Design review of the part built by this model. Coordinates are the model's own, in mm. Face numbers are marked on the shaded views. A direction names the side the tool comes from. Give positions to 0.01 mm unless a question says otherwise; leave off trailing zeros. Order: outer loops, then holes, each group sorted by start corner. A loop starts at its lowest first (then second) coordinate and runs counter-clockwise, first axis right, second up. Notation, with made-up numbers: (50.5, 27) -> (89.5, 27) arc R26 ccw to (89.5, 49) -> close; hole circle Ø9 at (32.5, 26.5). An arc over 180 degrees is marked (long way). One line per item, written item: value. Start each with the question number.
1) Tool access review of the marked faces 1 and 2: name each direction out of +Z, -Z, +X, -X, +Y, -Y from which nothing blocks a thin tool from reaching the whole face with its end or side.
2) Consider section A-A (y = 1.5). State the section outline as (x, z) points.
3) Consider section B-B (y = 6.5). State the section outline as (x, z) points, plus the area to 3 significant figures.
4) For pin 1 (3 mm diameter, centred on y = 5, z = -10.5, fed in from -X); pin 2 (3 mm diameter, centred on y = 3, z = -8, fed in from -X), all flat-tipped, find the tip position at first contact; note any pin that passes through.
5) The part is to be moulded in two halves that separate along X. For the marked faces 3, 4, 5 and 6, say which applies: released by +X, released by -X, zero draft, split by the parting line, or undercut.
6) Wall thickness on line 1 along Y through (x, z) = (-53.5, -10.25); line 2 along Y through (x, z) = (-57.25, -22.5); line 3 along Z through (x, y) = (-52.75, 1.75): over which ranges is each line inside the solid? List them lowest first. Write a range as from..to.
from build123d import *

# Parameters (mm, degrees)
SZKIC1_R                    = 9
SZKIC1_R_2                  = 5.477333333
DODANIE_WYCI_GNI_CIE1_DEPTH = 8
SZKIC1_3_R                  = 11
SZKIC1_3_R_2                = 9
DODANIE_WYCI_GNI_CIE2_DEPTH = 7
SZKIC1_4_R                  = 11.95
SZKIC1_4_R_2                = 11
DODANIE_WYCI_GNI_CIE3_DEPTH = 3
DODANIE_WYCI_GNI_CIE4_START = -3
SZKIC1_5_R                  = 11.95
SZKIC1_5_R_2                = 1.65
SZKIC1_5_R_3                = 11
SZKIC1_5_R_4                = 9
SZKIC1_5_R_5                = 5.477333333
DODANIE_WYCI_GNI_CIE4_DEPTH = 3
SZKIC2_R                    = 8.25
WYTNIJ_WYCI_GNI_CIE1_DEPTH  = 5
SFAZOWANIE1_SIZE            = 1.2
DODANIE_WYCI_GNI_CIE5_START = 17
SZKIC3_R                    = 1.65
DODANIE_WYCI_GNI_CIE5_DEPTH = 17
ZAOKR_GLENIE1_R             = 10
ZAOKR_GLENIE2_R             = 4
SFAZOWANIE2_SIZE            = 2
WYTNIJ_WYCI_GNI_CIE3_DEPTH  = 81.474279011


# Some blends are built 0.0001 mm under size
with BuildPart() as part:
    # Szkic1 → Dodanie-wyciągnięcie1 (new body)
    with BuildSketch(Plane(origin=(0, 0, 0), x_dir=(1, 0, 0), z_dir=(0, 1, 0))):
        with Locations(Location((-48.017326928, 15.231452718, 0), (0, 0, 270))):
            Circle(SZKIC1_R)
        with Locations(Location((-48.017326928, 15.231452718, 0), (0, 0, 270))):
            Circle(SZKIC1_R_2, mode=Mode.SUBTRACT)
    extrude(amount=DODANIE_WYCI_GNI_CIE1_DEPTH)

    # Szkic1<3> → Dodanie-wyciągnięcie2 (add)
    with BuildSketch(Plane(origin=(0, 0, 0), x_dir=(1, 0, 0), z_dir=(0, 1, 0))):
        with Locations(Location((-48.017326928, 15.231452718, 0), (0, 0, 270))):
            Circle(SZKIC1_3_R)
        with Locations(Location((-48.017326928, 15.231452718, 0), (0, 0, 270))):
            Circle(SZKIC1_3_R_2, mode=Mode.SUBTRACT)
    extrude(amount=DODANIE_WYCI_GNI_CIE2_DEPTH)

    # Szkic1<4> → Dodanie-wyciągnięcie3 (add)
    with BuildSketch(Plane(origin=(0, 0, 0), x_dir=(1, 0, 0), z_dir=(0, 1, 0))):
        with Locations(Location((-48.017326928, 15.231452718, 0), (0, 0, 270))):
            Circle(SZKIC1_4_R)
        with Locations(Location((-48.017326928, 15.231452718, 0), (0, 0, 270))):
            Circle(SZKIC1_4_R_2, mode=Mode.SUBTRACT)
    extrude(amount=DODANIE_WYCI_GNI_CIE3_DEPTH)

    # Szkic1<5> → Dodanie-wyciągnięcie4 (add)
    # profile 1 of 4: a face of its own
    with BuildSketch(Plane(origin=(0, 0, 0), x_dir=(1, 0, 0), z_dir=(0, 1, 0)).offset(DODANIE_WYCI_GNI_CIE4_START)):
        with BuildLine():
            Line((-69.017326928, 26.22592553), (-69.017326928, 4.236979905))
            ThreePointArc((-69.017326928, 4.236979905), (-67.978820752, -1.151729035), (-65.012060165, -5.768547282))
            Line((-65.012060165, -5.768547282), (-50.017326928, -5.768547282))
            Line((-50.017326928, -5.768547282), (-30.833560744, -5.768547282))
            Line((-30.833560744, -5.768547282), (-26.817326928, -1.752313466))
            Line((-26.817326928, -1.752313466), (-26.817326928, 32.215218902))
            Line((-26.817326928, 32.215218902), (-30.833560744, 36.231452718))
            Line((-30.833560744, 36.231452718), (-50.017326928, 36.231452718))
            Line((-50.017326928, 36.231452718), (-65.012060165, 36.231452718))
            ThreePointArc((-65.012060165, 36.231452718), (-67.978820752, 31.61463447), (-69.017326928, 26.22592553))
        make_face()
        with Locations(Location((-48.017326928, 15.231452718, 0), (0, 0, 270))):
            Circle(SZKIC1_5_R, mode=Mode.SUBTRACT)
        with Locations(Location((-63.517326928, -0.268547282, 0), (0, 0, 270))):
            Circle(SZKIC1_5_R_2, mode=Mode.SUBTRACT)
        with Locations(Location((-32.517326928, -0.268547282, 0), (0, 0, 270))):
            Circle(SZKIC1_5_R_2, mode=Mode.SUBTRACT)
        with Locations(Location((-32.517326928, 30.731452718, 0), (0, 0, 270))):
            Circle(SZKIC1_5_R_2, mode=Mode.SUBTRACT)
        with Locations(Location((-63.517326928, 30.731452718, 0), (0, 0, 270))):
            Circle(SZKIC1_5_R_2, mode=Mode.SUBTRACT)
    # profile 2 of 4: a face of its own
    with BuildSketch(Plane(origin=(0, 0, 0), x_dir=(1, 0, 0), z_dir=(0, 1, 0)).offset(DODANIE_WYCI_GNI_CIE4_START)):
        with Locations(Location((-48.017326928, 15.231452718, 0), (0, 0, 270))):
            Circle(SZKIC1_5_R)
        with Locations(Location((-48.017326928, 15.231452718, 0), (0, 0, 270))):
            Circle(SZKIC1_5_R_3, mode=Mode.SUBTRACT)
    # profile 3 of 4: a face of its own
    with BuildSketch(Plane(origin=(0, 0, 0), x_dir=(1, 0, 0), z_dir=(0, 1, 0)).offset(DODANIE_WYCI_GNI_CIE4_START)):
        with Locations(Location((-48.017326928, 15.231452718, 0), (0, 0, 270))):
            Circle(SZKIC1_5_R_3)
        with Locations(Location((-48.017326928, 15.231452718, 0), (0, 0, 270))):
            Circle(SZKIC1_5_R_4, mode=Mode.SUBTRACT)
    # profile 4 of 4: a face of its own
    with BuildSketch(Plane(origin=(0, 0, 0), x_dir=(1, 0, 0), z_dir=(0, 1, 0)).offset(DODANIE_WYCI_GNI_CIE4_START)):
        with Locations(Location((-48.017326928, 15.231452718, 0), (0, 0, 270))):
            Circle(SZKIC1_5_R_4)
        with Locations(Location((-48.017326928, 15.231452718, 0), (0, 0, 270))):
            Circle(SZKIC1_5_R_5, mode=Mode.SUBTRACT)
    extrude(amount=DODANIE_WYCI_GNI_CIE4_DEPTH)

    # Szkic2 → Wytnij-wyciągnięcie1 (cut)
    with BuildSketch(Plane.XZ.offset(3)):
        with Locations(Location((-48.017326928, -15.231452718, 0), (0, 0, 270))):
            Circle(SZKIC2_R)
    extrude(amount=-WYTNIJ_WYCI_GNI_CIE1_DEPTH, mode=Mode.SUBTRACT)

    # Sfazowanie1
    # the kernel refuses this chamfer: 1.2 mm, written as the material it takes off along each edge
    with BuildSketch(Plane(origin=(-48.017326928, 3, -15.231452718), x_dir=(0, 0, 1), z_dir=(-1, 0, 0))) as sfazowanie1_piece_1_section:
        Polygon((11.95 - SFAZOWANIE1_SIZE, 0), (11.95, -SFAZOWANIE1_SIZE), (11.95, 0), align=None)
    sfazowanie1_piece_1 = revolve(axis=Axis((-48.017326928, 3, -15.231452718), (0, 1, 0)), mode=Mode.PRIVATE)
    sfazowanie1_piece_1 = sfazowanie1_piece_1 - Plane(origin=(-48.017326928, 2.284838346, -15.231452718), x_dir=(0, 0, 1), z_dir=(0, -1, 0)) * Cylinder(11, 48, mode=Mode.PRIVATE)
    add(sfazowanie1_piece_1, mode=Mode.SUBTRACT)

    # Szkic3 → Dodanie-wyciągnięcie5 (add)
    with BuildSketch(Plane.XZ.offset(3).offset(DODANIE_WYCI_GNI_CIE5_START)):
        with BuildLine():
            Line((-69.017326928, -26.22592553), (-36.817326928, -26.22592553))
            Line((-36.817326928, -26.22592553), (-36.817326928, -4.236979905))
            Line((-36.817326928, -4.236979905), (-69.017326928, -4.236979905))
            ThreePointArc((-69.017326928, -4.236979905), (-67.978820752, 1.151729035), (-65.012060165, 5.768547282))
            Line((-65.012060165, 5.768547282), (-30.833560744, 5.768547282))
            Line((-30.833560744, 5.768547282), (-26.817326928, 1.752313466))
            Line((-26.817326928, 1.752313466), (-26.817326928, -32.215218902))
            Line((-26.817326928, -32.215218902), (-30.833560744, -36.231452718))
            Line((-30.833560744, -36.231452718), (-65.012060165, -36.231452718))
            ThreePointArc((-65.012060165, -36.231452718), (-67.978820752, -31.61463447), (-69.017326928, -26.22592553))
        make_face()
        with Locations(Location((-63.517326928, 0.268547282, 0), (0, 0, 90))):
            Circle(SZKIC3_R, mode=Mode.SUBTRACT)
        with Locations(Location((-32.517326928, 0.268547282, 0), (0, 0, 90))):
            Circle(SZKIC3_R, mode=Mode.SUBTRACT)
        with Locations(Location((-32.517326928, -30.731452718, 0), (0, 0, 90))):
            Circle(SZKIC3_R, mode=Mode.SUBTRACT)
        with Locations(Location((-63.517326928, -30.731452718, 0), (0, 0, 90))):
            Circle(SZKIC3_R, mode=Mode.SUBTRACT)
    extrude(amount=-DODANIE_WYCI_GNI_CIE5_DEPTH)

    # Zaokrąglenie1
    zaokr_glenie1_edges = [part.edges().sort_by_distance(p)[0] for p in [
        (-36.817326928, -11.5, -4.236979905),
        (-36.817326928, -11.5, -26.22592553),
    ]]
    fillet(zaokr_glenie1_edges, radius=ZAOKR_GLENIE1_R)

    # Zaokrąglenie2
    zaokr_glenie2_edges = [part.edges().sort_by_distance(p)[0] for p in [
        (-65.012060165, -10, -36.231452718),
        (-30.833560744, -10, -36.231452718),
        (-26.817326928, -10, -32.215218902),
        (-26.817326928, -10, 1.752313466),
        (-30.833560744, -10, 5.768547282),
        (-65.012060165, -10, 5.768547282),
        (-69.017326928, -11.5, -26.22592553),
        (-69.017326928, -11.5, -4.236979905),
    ]]
    fillet(zaokr_glenie2_edges, radius=ZAOKR_GLENIE2_R)

    # Sfazowanie2
    sfazowanie2_edges = [part.edges().sort_by_distance(p)[0] for p in [
        (-48.017326928, 7, -26.231452718),
    ]]
    chamfer(sfazowanie2_edges, length=SFAZOWANIE2_SIZE - 0.0001)  # a hair under: the kernel refuses the full size

    # Szkic5 → Wytnij-wyciągnięcie3 (cut, through all)
    with BuildSketch(Plane(origin=(0, 0, 0), x_dir=(1, 0, 0), z_dir=(0, 1, 0))):
        with BuildLine():
            Line((-63.130319625, -5.768547282), (-32.490414994, -5.768547282))
            ThreePointArc((-32.490414994, -5.768547282), (-30.959681264, -5.464065412), (-29.661987869, -4.596974407))
            Line((-29.661987869, -4.596974407), (-27.988899803, -2.923886342))
            ThreePointArc((-27.988899803, -2.923886342), (-27.121808798, -1.626192946), (-26.817326928, -0.095459217))
            Line((-26.817326928, -0.095459217), (-26.817326928, 30.558364652))
            ThreePointArc((-26.817326928, 30.558364652), (-27.121808798, 32.089098382), (-27.988899803, 33.386791777))
            Line((-27.988899803, 33.386791777), (-29.661987869, 35.059879842))
            ThreePointArc((-29.661987869, 35.059879842), (-30.959681264, 35.926970848), (-32.490414994, 36.231452718))
            Line((-32.490414994, 36.231452718), (-63.130319625, 36.231452718))
            ThreePointArc((-63.130319625, 36.231452718), (-64.980822324, 35.777667568), (-66.411459701, 34.519272599))
            ThreePointArc((-66.411459701, 34.519272599), (-68.350528387, 30.572480189), (-69.017326928, 26.22592553))
            Line((-69.017326928, 26.22592553), (-69.017326928, 4.236979905))
            ThreePointArc((-69.017326928, 4.236979905), (-68.350528387, -0.109574754), (-66.411459701, -4.056367163))
            ThreePointArc((-66.411459701, -4.056367163), (-64.980822324, -5.314762132), (-63.130319625, -5.768547282))
        make_face()
    extrude(amount=-WYTNIJ_WYCI_GNI_CIE3_DEPTH, mode=Mode.SUBTRACT)


solid = part.part
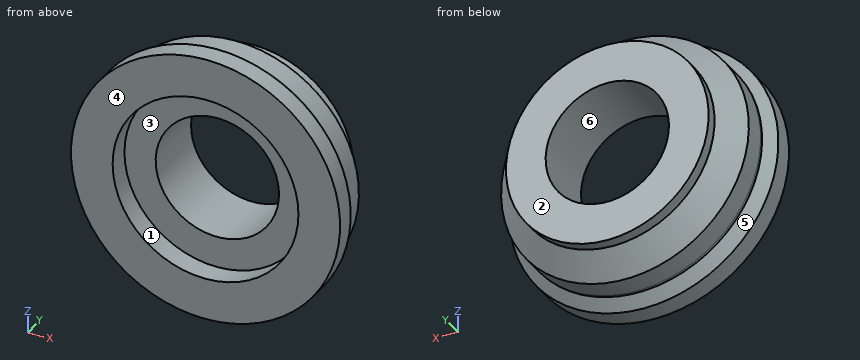
Checked values:
1. face 1: -Y
1. face 2: +Z, -Z, +X, -X, +Y
2. outline: circle Ø23.9 at (-48.02, -15.23); hole circle Ø16.5 at (-48.02, -15.23)
3. outline: circle Ø19 at (-48.02, -15.23); hole circle Ø10.95 at (-48.02, -15.23)
3. area: 189 mm^2
4. pin 1: stops at x = -58.53
4. pin 2: stops at x = -58.15
5. face 3: undercut
5. face 4: zero draft
5. face 5: split by the parting line
5. face 6: undercut
6. line 1: y = 2..8
6. line 2: y = 0..2
6. line 3: z = -26.2..-21.99, -8.47..-4.26
